from build123d import *

# Parameters (mm, degrees)
F1_DEPTH = 38.1


with BuildPart() as f1:
    # F0 (on Front) → F1 (new body)
    with BuildSketch(Plane.XZ):
        Polygon((351.952724098, 609.6), (-351.952724098, 609.6), (-703.905448196, 0), (-351.952724098, -609.6), (351.952724098, -609.6), (703.905448196, 0), align=None)
        Polygon((12.7, 584.2), (337.2880272606, 584.2), (499.5820408909, 303.0985226281), (512.2820408909, 281.1014773719), (674.5760545212, 0), (512.2820408909, -281.1014773719), (499.5820408909, -303.0985226281), (337.2880272606, -584.2), (12.7, -584.2), (-12.7, -584.2), (-337.2880272606, -584.2), (-499.5820408909, -303.0985226281), (-512.2820408909, -281.1014773719), (-674.5760545212, 0), (-512.2820408909, 281.1014773719), (-499.5820408909, 303.0985226281), (-449.9381191901, 389.0843173008), (-337.2880272606, 584.2), (-12.7, 584.2), align=None, mode=Mode.SUBTRACT)
        with BuildLine():
            Line((12.7, 380.7882745043), (12.7, 584.2))
            Line((12.7, 584.2), (-12.7, 584.2))
            Line((-12.7, 584.2), (-12.7, 380.7882745043))
            ThreePointArc((-12.7, 380.7882745043), (0, 381), (12.7, 380.7882745043))
        make_face()
        with BuildLine():
            ThreePointArc((-336.122319184, 179.3956146241), (-329.9556788419, 190.5), (-323.422319184, 201.3926598802))
            Line((-323.422319184, 201.3926598802), (-499.5820408909, 303.0985226281))
            Line((-499.5820408909, 303.0985226281), (-512.2820408909, 281.1014773719))
            Line((-512.2820408909, 281.1014773719), (-336.122319184, 179.3956146241))
        make_face()
        with BuildLine():
            Line((512.2820408909, 281.1014773719), (499.5820408909, 303.0985226281))
            Line((499.5820408909, 303.0985226281), (323.422319184, 201.3926598802))
            ThreePointArc((323.422319184, 201.3926598802), (329.9556788419, 190.5), (336.122319184, 179.3956146241))
            Line((336.122319184, 179.3956146241), (512.2820408909, 281.1014773719))
        make_face()
        with BuildLine():
            Line((499.5820408909, -303.0985226281), (512.2820408909, -281.1014773719))
            Line((512.2820408909, -281.1014773719), (336.122319184, -179.3956146241))
            ThreePointArc((336.122319184, -179.3956146241), (329.9556788419, -190.5), (323.422319184, -201.3926598802))
            Line((323.422319184, -201.3926598802), (499.5820408909, -303.0985226281))
        make_face()
        with BuildLine():
            Line((-12.7, -584.2), (12.7, -584.2))
            Line((12.7, -584.2), (12.7, -380.7882745043))
            ThreePointArc((12.7, -380.7882745043), (0, -381), (-12.7, -380.7882745043))
            Line((-12.7, -380.7882745043), (-12.7, -584.2))
        make_face()
        with BuildLine():
            ThreePointArc((-323.422319184, -201.3926598802), (-329.9556788419, -190.5), (-336.122319184, -179.3956146241))
            Line((-336.122319184, -179.3956146241), (-512.2820408909, -281.1014773719))
            Line((-512.2820408909, -281.1014773719), (-499.5820408909, -303.0985226281))
            Line((-499.5820408909, -303.0985226281), (-323.422319184, -201.3926598802))
        make_face()
    extrude(amount=F1_DEPTH)


solid = f1.part
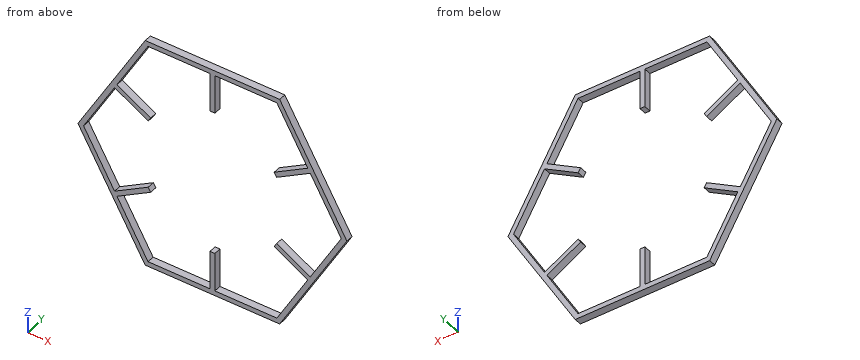
Can you work these out from the model? Positions are in its coordinate system, mm. Coordinates: 2 decimals unless noted, no trailing zeros. Loops run counter-clockwise (first coordinate to the right, second up) from the corner with the lowest first, then second, coordinate; pieces in that order, holes last. Notation, with made-up numbers: M 53,-36 L 69,-36 A20 ccw 69,-10 Z; hole C -18,59 d1. An arc over 180 degrees is marked long. Return JSON: item names as keys, results as strings. Group by question number.
Item 1: Imagine slicing it at D-D (x = 602.5). Please give me the cut outline in (y, z), and give its area (3 significant figures).
Item 2: Imagine slicing it at B-B (x = 109). Please give me the cut outline in (y, z).
Item 3: If I drill on L1, parallel to Z at x = -234.5, y = -2; L2, parallel to Z at x = -408.5, y = -6; L3, parallel to Z at x = -390, y = -25, over which ranges is the centre line in solid material (lowest first)? Write a range as from..to.
Item 4: I'm going to push flat-ended pins straight in: pin 1 Ø3 at (y, z) = (-34, 449.5) entering from +X; pin 2 Ø11.5 at (y, z) = (-24.5, -511) entering from -X; pin 3 Ø5 at (y, z) = (-33.5, -233.5) entering from +X. Where does each tip first touch, or does it pass through?
Item 5: Imagine slicing it at C-C (z = -520.5). Please give me the cut outline in (x, y), and give its area (3 significant figures).
Item 6: Imagine slicing it at A-A (x = -408). Please give me the cut outline in (y, z), and give its area (3 significant figures).
Verdict:
{
 "1": {"outline": "M -38.1,-175.64 L 0,-175.64 L 0,-124.84 L -38.1,-124.84 Z; M -38.1,124.84 L 0,124.84 L 0,175.64 L -38.1,175.64 Z", "area": "3,870 mm^2"},
 "2": {"outline": "M -38.1,-609.6 L 0,-609.6 L 0,-584.2 L -38.1,-584.2 Z; M -38.1,584.2 L 0,584.2 L 0,609.6 L -38.1,609.6 Z"},
 "3": {"L1": "z = -609.6..-584.2, 584.2..609.6", "L2": "z = -511.66..-460.86, -250.51..-221.18, 221.18..250.51, 460.86..511.66", "L3": "z = -543.7..-492.9, -239.83..-210.5, 210.5..239.83, 492.9..543.7"},
 "4": {"pin 1": "stops at x = 445.25", "pin 2": "stops at x = -412.2", "pin 3": "stops at x = 570.54"},
 "5": {"outline": "M -403.39,-38.1 L -374.07,-38.1 L -374.07,0 L -403.39,0 Z; M -12.7,-38.1 L 12.7,-38.1 L 12.7,0 L -12.7,0 Z; M 374.07,-38.1 L 403.39,-38.1 L 403.39,0 L 374.07,0 Z", "area": "3,200 mm^2"},
 "6": {"outline": "M -38.1,-512.52 L 0,-512.52 L 0,-461.72 L -38.1,-461.72 Z; M -38.1,-250.22 L 0,-250.22 L 0,-220.89 L -38.1,-220.89 Z; M -38.1,220.89 L 0,220.89 L 0,250.22 L -38.1,250.22 Z; M -38.1,461.72 L 0,461.72 L 0,512.52 L -38.1,512.52 Z", "area": "6,110 mm^2"}
}
